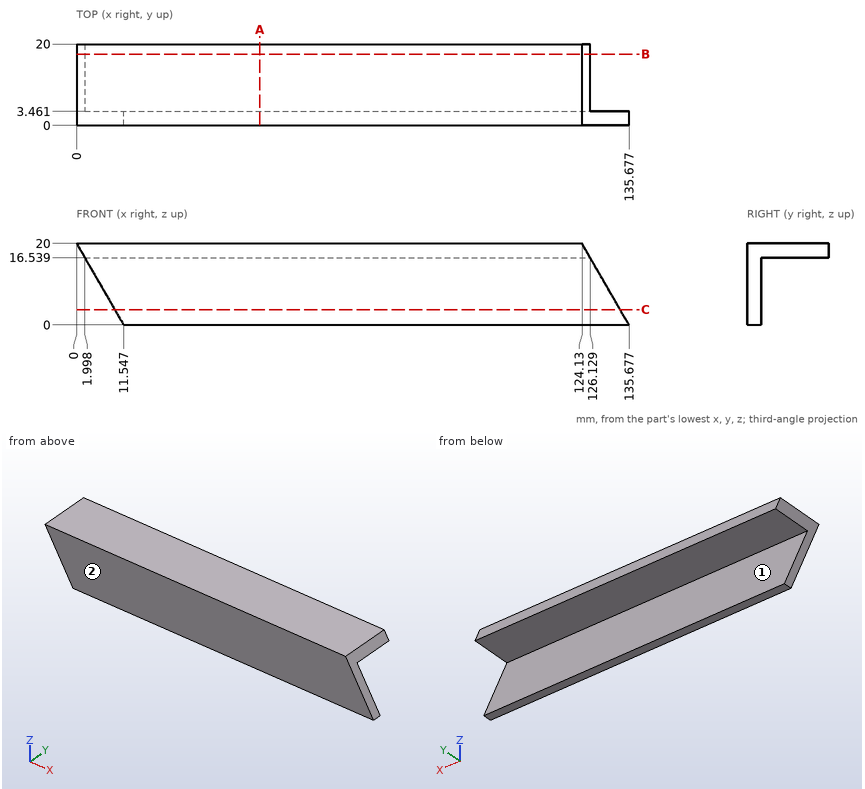
For this review, use the dimensioned drawing (mm, ordinates from the lowest corner) and the shaded views. A direction names the side the tool comes from. Give positions to 0.01 mm unless a question says otherwise; leave off trailing zeros. Write each loop counter-clockwise with the first axis right and the second up, starting at its lowest first coordinate (ties: lowest second). Pieces come first, ordered by that corner, then holes. Notation, with made-up numbers: M 65,74 L 93,74 A21 cw 93,106 Z; hole C 89,43.5 d10. An arc over 180 degrees is marked long. Answer as a JSON object with one key per item and string values. Group by question number.
1) Clearance check with flat-ended pins moving along their axes: pin 1 Ø1.5 at (x, z) = (69.5, 17.5) entering from -Y; pin 2 Ø8 at (x, y) = (45, 13.5) entering from -Z; pin 3 Ø8 at (y, z) = (14, 16) entering from +X; pin 4 Ø5 at (x, z) = (68, 10) entering from +Y. State where each tip first meets the part, or that it passes through.
2) We need section C-C (z = 3.75). Give the boundary of the cut face in (x, y).
3) For line 1 along Z through (x, y) = (43.5, 10); line 2 along Y through (x, z) = (63, 7.75); line 3 along X through (y, z) = (2, 12), list the stretches that pass through material, from the lowest coordinate up.
4) Tool access review of the marked faces 1 and 2: name each direction out of +Z, -Z, +X, -X, +Y, -Y from which nothing blocks a thin tool from reaching the whole face with its end or side.
5) We need section B-B (y = 17.5). Give the boundary of the cut face in (x, z).
6) We need section A-A (x = 45). Give the boundary of the cut face in (y, z).
Answer key:
{
 "1": {"pin 1": "stops at y = 0", "pin 2": "stops at z = 16.54", "pin 3": "stops at x = 126.13", "pin 4": "stops at y = 3.46"},
 "2": {"outline": "M 9.38,0 L 133.51,0 L 133.51,3.46 L 9.38,3.46 Z"},
 "3": {"line 1": "z = 16.54 to 20", "line 2": "y = 0 to 3.46", "line 3": "x = 4.62 to 128.75"},
 "4": {"face 1": "-Z, +X, -X, +Y", "face 2": "+Z, -Z, +X, -X, -Y"},
 "5": {"outline": "M 0,20 L 2,16.54 L 126.13,16.54 L 124.13,20 Z"},
 "6": {"outline": "M 0,0 L 3.46,0 L 3.46,16.54 L 20,16.54 L 20,20 L 0,20 Z"}
}
